```python
from build123d import *

# Parameters (mm, degrees)
F0_W     = 50
F0_H     = 8
F1_DEPTH = 25
F2_R     = 3.99999
F3_R     = 5


# Not quite as in the source:
# - a fillet or chamfer is up to 0.001 mm smaller than in the source, because OpenCascade refuses the exact size


with BuildPart() as f1:
    # F0 (on Front) → F1 (new body)
    with BuildSketch(Plane.XZ):
        with BuildLine():
            ThreePointArc((-33.1246824974, 28.5893382254), (-21.8780417926, 8.1356985419), (0, 0))
            Line((0, 0), (0, 9.0772153518))
            ThreePointArc((0, 9.0772153518), (-15.8507153639, 14.5046379043), (-24.9239347471, 28.5893382254))
            ThreePointArc((-24.9239347471, 28.5893382254), (-29.0243086222, 33.6818376736), (-33.1246824974, 28.5893382254))
        make_face()
        with Locations((33, 42)):
            Rectangle(F0_W, F0_H)
        Polygon((57.6595105231, 10.0428396836), (8, 8), (57.743546671, 8), align=None)
        Polygon((0, 9.0772153518), (0, 0), (8, 0), (8, 8), (8, 38), (8, 46), (0, 46), align=None)
        Polygon((8, 8), (8, 0), (58, 1.7658608791), (57.743546671, 8), align=None)
    extrude(amount=F1_DEPTH)

    # F2 (radius 4 in the source; OpenCascade refuses exactly that, so slightly less here)
    f2_edges = [f1.edges().sort_by_distance(p)[0] for p in [
        (58, -12.5, 46),
        (58, -12.5, 38),
        (57.659511, -12.5, 10.04284),
        (58, -12.5, 1.765861),
    ]]
    fillet(f2_edges, radius=F2_R)

    # F3
    f3_edges = [f1.edges().sort_by_distance(p)[0] for p in [
        (-15.850715, -25, 14.504638),
        (-15.850715, 0, 14.504638),
        (0, -12.5, 46),
    ]]
    fillet(f3_edges, radius=F3_R)


solid = f1.part
```
Model file for the job. Use its own axes, mm. A direction names the side the tool comes from. Give positions to 0.01 mm unless a question says otherwise; leave off trailing zeros. Write each loop counter-clockwise with the first axis right and the second up, starting at its lowest first coordinate (ties: lowest second). Pieces come first, ordered by that corner, then holes. Notation, with made-up numbers: (-0.5, 12.25) - (37.5, 12.25) arc R19 ccw to (37.5, 34.25) - close; hole circle Ø7 at (-38.5, 87). An arc over 180 degrees is marked (long way). One line per question, with ' | ' between items. Start each with the question number.
(1) Slice it at C-C on x = 1. Write the cut outline in (y, z), plus the area to 3 significant figures.
(2) Slice it at B-B on x = 18. Write the cut outline in (y, z), plus the area to 3 significant figures.
(3) Slice it at A-A on z = 31.5. Write the cut outline in (x, y).
(4) Two-plate mould, pull along X, no slides. Class faces 1 (the face through (56.797, -12.675, 39.141)), 2 (the face through (0, -12, 23)), 3 (the face through (1, -13, 44)): +X half, -X half, draft (parallel to the pull), parting line (faces both ways), or undercut.
(5) Wall check: line 1 along Z through (x, y) = (40.5, -9); line 2 along Z through (x, y) = (18, -23); line 3 along X through (y, z) = (-14.5, 23). Give the ranges that are in metal, low to high. Write a range as from..to.
(6) 3-axis set-ups, long thin cutter, end or side, ignore diameter. For faces 4 (the face through (31.151, -12.325, 8.952)), 5 (the face through (31, -12, 38)), 6 (the face through (56.859, -12.675, 44.797)): which of +Z, -Z, +X, -X, +Y, -Y reach the whole face in a straight line?
(7) Slice it at D-D on z = 39.5. Write the cut outline in (x, y), plus the area to 3 significant figures.
(8) Pin check, flat tips, straight feed: P1, Ø2, axis at y = -17, z = 19, coming from the +X side; P2, Ø12, axis at y = -14.5, z = 21.5, coming from the -X side; P3, Ø5, axis at x = -10.5, y = -5.5, coming from the +Z side. Stop position of each tip, or through.
Results below:
1) outline: (-25, 0) - (0, 0) - (0, 44) - (-25, 44) - close | area: 1,100 mm^2
2) outline: (-25, 0.35) - (0, 0.35) - (0, 8.41) - (-25, 8.41) - close; (-25, 38) - (0, 38) - (0, 46) - (-25, 46) - close | area: 401 mm^2
3) outline: (-32.71, -25) - (-25.34, -25) - (-25.34, 0) - (-32.71, 0) - close; (0, -25) - (8, -25) - (8, 0) - (0, 0) - close
4) face 1: +X half | face 2: undercut | face 3: -X half
5) line 1: 1.15..9.34, 38..46 | line 2: 0.35..8.41, 38..46 | line 3: -31.8..-22.85, 0..8
6) face 4: +Y, -Y | face 5: +X, +Y, -Y | face 6: +Z, +X, +Y, -Y
7) outline: (0, -25) - (57.12, -25) - (57.12, 0) - (0, 0) - close | area: 1,430 mm^2
8) P1: x = 8 | P2: x = -32.95 | P3: z = 12.57
